Model file for the job. Use its own axes, mm. Coordinates: 2 decimals unless noted, no trailing zeros. Write each loop counter-clockwise with the first axis right and the second up, starting at its lowest first coordinate (ties: lowest second). Pieces come first, ordered by that corner, then holes. Notation, with made-up numbers: M -25,26 L 8,26 A19 ccw 8,32 Z; hole C 24,-9.5 d11. An arc over 180 degrees is marked long. Put each result on its own line as item: value. Start each with the question number.
Q1. Cut at D-D (y = -30). Write the cut outline in (x, z) (3 decimals), then the cut area to 3 significant figures.
Q2. Cut at C-C (x = 131). Write the cut outline in (y, z) (3 decimals).
Q3. Cut at A-A (x = -112). Write the cut outline in (y, z) (3 decimals), then the cut area to 3 significant figures.
Q4. Cut at B-B (z = 4.75). Give the number of separate pieces and of enclosed holes in the cut face, then the cut area to 3 significant figures.
Q5. Drop flat-ended pins along their axis: pin 1 (1.7 mm diameter, centred on y = -47.5, z = 3.5, fed in from +X); pin 2 (13.5 mm diameter, centred on x = 0, y = 81.81, fed in from -Z); pin 3 (1.7 mm diameter, centred on y = 93, z = 5.5, fed in from -X); pin 4 (4.5 mm diameter, centred on y = 92, z = 5, fed in from +X). Give the stop position or say it passes through.
Q6. Drill centre lines: line 1 along X through (y, z) = (-292.1, 2) (3 decimals); line 2 along Y through (x, z) = (0, 6.25); line 3 along Y through (x, z) = (-4, 2). Where is each one in solid material? Low to high.
Q7. Pull direction Y, two halves, no side cores. Call faces 1 (the cylindrical face through (171.003, 281.053, 4.829)), 2 (the cylindrical face through (-0.297, -66.263, 4.829)), 3 (the flat face through (2, -9, 9.525)), 4 (the cylindrical face through (-171.003, -307.331, 4.829)): pulls with the +Y half, pulls with the -Y half, needs draft (parallel to the pull), parting line crosses it, or undercut.
```python
from build123d import *

# Parameters (mm, degrees)
BOSS_EXTRUDE1_DEPTH            = 9.525
V_0_377_DIAMETER_SLOT1_DEPTH   = 9.525
FILLET1_R                      = 12.7
SKETCH6_R                      = 8.382
CUT_EXTRUDE1_DEPTH             = 357.929879318
F_5_16_0_3125_DIAMETER_HOLE1_D = 7.9375
SKETCH14_W                     = 349.25
SKETCH14_H                     = 26.277954941
CUT_EXTRUDE3_DEPTH             = 357.929879318
FILLET2_R                      = 12.7


# Read off the part's stored shape, not the designer's step: V (0.377) Diameter Slot1
with BuildPart() as part:
    # Sketch1 → Boss-Extrude1 (new body)
    with BuildSketch(Plane.XY):
        with BuildLine():
            Line((-174.625, 151.522045059), (-174.625, 311.15))
            Line((-174.625, 311.15), (174.625, 311.15))
            Line((174.625, 311.15), (174.625, 151.522045059))
            ThreePointArc((174.625, 151.522045059), (66.675, -31.75), (174.625, -215.022045059))
            Line((174.625, -215.022045059), (174.625, -311.15))
            Line((174.625, -311.15), (-174.625, -311.15))
            Line((-174.625, -311.15), (-174.625, -215.022045059))
            ThreePointArc((-174.625, -215.022045059), (-66.675, -31.75), (-174.625, 151.522045059))
        make_face()
    extrude(amount=BOSS_EXTRUDE1_DEPTH)

    # V (0.377) Diameter Slot1 outline → V (0.377) Diameter Slot1 (cut)
    with BuildSketch(Plane.XY):
        with BuildLine():
            Line((4.7879, -57.8866), (4.7879, -45.2374))
            ThreePointArc((4.7879, -45.2374), (0, -40.4495), (-4.7879, -45.2374))
            Line((-4.7879, -45.2374), (-4.7879, -57.8866))
            ThreePointArc((-4.7879, -57.8866), (0, -62.6745), (4.7879, -57.8866))
        make_face()
        with BuildLine():
            ThreePointArc((4.7879, 94.4626), (0, 99.2505), (-4.7879, 94.4626))
            Line((-4.7879, 94.4626), (-4.7879, 81.8134))
            ThreePointArc((-4.7879, 81.8134), (0, 77.0255), (4.7879, 81.8134))
            Line((4.7879, 81.8134), (4.7879, 94.4626))
        make_face()
        with BuildLine():
            ThreePointArc((4.7879, -184.9374), (0, -180.1495), (-4.7879, -184.9374))
            Line((-4.7879, -184.9374), (-4.7879, -197.5866))
            ThreePointArc((-4.7879, -197.5866), (0, -202.3745), (4.7879, -197.5866))
            Line((4.7879, -197.5866), (4.7879, -184.9374))
        make_face()
    extrude(amount=V_0_377_DIAMETER_SLOT1_DEPTH, mode=Mode.SUBTRACT)

    # Fillet1
    fillet1_edges = [part.edges().sort_by_distance(p)[0] for p in [
        (174.625, -311.15, 4.7625),
        (-174.625, -311.15, 4.7625),
    ]]
    fillet(fillet1_edges, radius=FILLET1_R)

    # Sketch6 → Cut-Extrude1 (cut, through all)
    with BuildSketch(Plane.XY.offset(9.525)):
        with Locations((0, -197.5866)):
            Circle(SKETCH6_R)
        with Locations((0, 81.8134)):
            Circle(SKETCH6_R)
        with Locations((0, -57.8866)):
            Circle(SKETCH6_R)
    extrude(amount=-CUT_EXTRUDE1_DEPTH, mode=Mode.SUBTRACT)

    # 5/16 (0.3125) Diameter Hole1 (through all)
    with Locations(Plane(origin=(0, 0, 0), x_dir=(-1, 0, 0), z_dir=(0, 0, -1))):
        with Locations((-85.725, 265.938), (85.725, 170.688), (85.725, 265.938), (-85.725, 170.688), (85.725, -234.95), (85.725, -292.1), (-85.725, -292.1), (-85.725, -234.95)):
            Hole(F_5_16_0_3125_DIAMETER_HOLE1_D / 2)

    # Sketch14 → Cut-Extrude3 (cut, through all)
    with BuildSketch(Plane(origin=(0, 0, 0), x_dir=(-1, 0, 0), z_dir=(0, 0, -1))):
        with Locations((0, 298.011022529)):
            Rectangle(SKETCH14_W, SKETCH14_H)
    extrude(amount=-CUT_EXTRUDE3_DEPTH, mode=Mode.SUBTRACT)

    # Fillet2
    fillet2_edges = [part.edges().sort_by_distance(p)[0] for p in [
        (174.625, 284.872045059, 4.7625),
        (-174.625, 284.872045059, 4.7625),
    ]]
    fillet(fillet2_edges, radius=FILLET2_R)


solid = part.part
```
Computed values:
1. outline: M -66.682,0 L 66.682,0 L 66.682,9.525 L -66.682,9.525 Z
1. area: 1,270 mm2
2. outline: M -311.15,0 L -182.816,0 L -182.816,9.525 L -311.15,9.525 Z; M 119.316,0 L 284.872,0 L 284.872,9.525 L 119.316,9.525 Z
3. outline: M -311.15,0 L -161.909,0 L -161.909,9.525 L -311.15,9.525 Z; M 98.409,0 L 284.872,0 L 284.872,9.525 L 98.409,9.525 Z
3. area: 3,200 mm2
4. separate pieces: 1
4. enclosed holes: 11
4. area: 150,000 mm2
5. pin 1: x = 67.33
5. pin 2: through
5. pin 3: x = -108.49
5. pin 4: x = 108.79
6. line 1: -174.625 to -89.694, -81.756 to 81.756, 89.694 to 174.625
6. line 2: -311.15 to -205.97, -180.15 to -66.27, -40.45 to 73.43, 99.25 to 284.87
6. line 3: -311.15 to -204.95, -182.31 to -65.25, -42.61 to 74.45, 97.09 to 284.87
7. face 1: pulls with the +Y half
7. face 2: undercut
7. face 3: needs draft
7. face 4: pulls with the -Y half
